Autodesk Inventor part; units mm, degrees
ref_plane "YZ Plane" through (0, 0, 0) normal (1, 0, 0) x (0, 1, 0)
ref_plane "XZ Plane" through (0, 0, 0) normal (0, 1, 0) x (-1, 0, 0)
ref_plane "XY Plane" through (0, 0, 0) normal (0, 0, 1) x (1, 0, 0)
sketch "Sketch1" plane through (0, 0, 0) normal (0, 0, 1) x (1, 0, 0)
  line L0 (0, 0) -> (25.4, 0)
  line L1 (25.4, 76.2) -> (0, 76.2)
  line L2 (0, 76.2) -> (0, 0)
  line L3 (25.4, 3.175) -> (3.175, 3.175)
  line L4 (3.175, 3.175) -> (3.175, 73.025)
  line L5 (3.175, 73.025) -> (25.4, 73.025)
  line L6 (25.4, 0) -> (25.4, 3.175)
  line L7 (25.4, 73.025) -> (25.4, 76.2)
  dimension "d0" = 76.2
  dimension "d1" = 25.4
  dimension "d2" = 3.175
  dimension "d3" = 3.175
  dimension "d4" = 3.175
extrude "Extrusion1" add sketch "Sketch1" along normal blind 685.8
sketch "Sketch2" plane through (0, 76.2, 0) normal (0, 1, 0) x (1, 0, 0)
  line L0 (0, -685.8) -> (25.4, -685.8)
  line L1 (25.4, 0) -> (25.4, -685.8)
  line L2 (25.4, 0) -> (0, 0)
  line L3 (0, 0) -> (0, -685.8)
  line L4 (0, -685.8) -> (25.4, -660.4)
  line L5 (0, 0) -> (25.4, -25.4)
  line L6 (3.175, -682.625) -> (3.175, -517.525)
  line L7 (3.175, -517.525) -> (25.4, -517.525)
  line L8 (3.175, -3.175) -> (3.175, -168.275)
  line L9 (3.175, -168.275) -> (25.4, -168.275)
  dimension "d7" = 45
  dimension "d8" = 3.175
  dimension "d9" = 165.1
  dimension "d10" = 165.1
extrude "Extrusion2" cut sketch "Sketch2" against normal through all contours L4 L1 L0 | L2 L1 L5
extrude "Extrusion3" cut sketch "Sketch2" against normal up to next contours L6 L7 L1 L4 | L5 L1 L9 L8
equation "\"d3\" = d2"
equation "\"d4\" = d2"
equation "\"d10\" = d9"
properties part number "frame U 1 by 3"
Can you work these out from the model? Positions are in its coordinate system, mm. A direction names the side the tool comes from. Round coordinates to 2 decimals unless told otherwise and drop trailing zeros. Order: outer loops, then holes, each group sorted by start corner. A loop starts at its lowest first (then second) coordinate and runs counter-clockwise, first axis right, second up. Notation, with made-up numbers: (80.25, 35) -> (101.25, 35) arc R27 cw to (101.25, 65) -> close; hole circle Ø11 at (47, 67). An arc over 180 degrees is marked (long way). Return JSON: item names as keys, results as strings. Group by question number.
1. If we section it at C-C, the plane y = 27.5: Write out the boundary of the cut face in (x, z) (3 decimals), then the cut area to 3 significant figures.
2. I need wall thicknesses on line 1 (Y direction, x = 12, z = 222.5) (3 decimals); line 2 (X direction, y = 33, z = 478) (3 decimals). Which ranges of each line are inside material? Lowest first, please. Write a range as [from, to].
3. We'd pull the mould along Y, two halves only. Please class faces 3 (the face through (3.175, 40, 348)), 4 (the face through (2, 30, 2)), 5 (the face through (13, 0, 338)): released by +Y, released by -Y, zero draft, split by the parting line, or undercut.
4. Which directions (+Z, -Z, +X, -X, +Y, -Y) give clear straight access to the entire face, cutting with the end or side of a thin tool? Please do faces 1 (the face through (14, 73.025, 340)), 2 (the face through (13, 76.2, 338)).
5. Will these pins go through, and if not, where does the flat tip stop? pin 1 (1.6 mm diameter, centred on x = 17.5, y = 75.5, fed in from -Z) (3 decimals); pin 2 (1.5 mm diameter, centred on y = 12, z = 74, fed in from +X) (3 decimals); pin 3 (3.5 mm diameter, centred on x = 10, y = 75, fed in from +Z) (3 decimals).
6. If we section it at D-D, the plane z = 193: Write out the boundary of the cut face in (x, y) (3 decimals), then the cut area to 3 significant figures.
7. If we section it at B-B, the plane z = 630: Write out the boundary of the cut face in (x, y) (3 decimals), then the cut area to 4 significant figures.
8. If we section it at A-A, the plane x = 20.75: Write out the boundary of the cut face in (y, z) (3 decimals), then the cut area to 3 significant figures.
Output values:
{
 "1": {"outline": "(0, 0) -> (3.175, 3.175) -> (3.175, 682.625) -> (0, 685.8) -> close", "area": "2,170 mm²"},
 "2": {"line 1": "[0, 3.175], [73.025, 76.2]", "line 2": "[0, 3.175]"},
 "3": {"face 3": "undercut", "face 4": "zero draft", "face 5": "released by -Y"},
 "4": {"face 1": "+Z, -Z, +X", "face 2": "+Z, -Z, +X, -X, +Y"},
 "5": {"pin 1": "z = 168.275", "pin 2": "x = 3.175", "pin 3": "z = 517.525"},
 "6": {"outline": "(0, 0) -> (25.4, 0) -> (25.4, 3.175) -> (3.175, 3.175) -> (3.175, 73.025) -> (25.4, 73.025) -> (25.4, 76.2) -> (0, 76.2) -> close", "area": "383 mm²"},
 "7": {"outline": "(0, 0) -> (25.4, 0) -> (25.4, 3.175) -> (3.175, 3.175) -> (3.175, 76.2) -> (0, 76.2) -> close", "area": "312.5 mm²"},
 "8": {"outline": "(0, 20.75) -> (3.175, 20.75) -> (3.175, 665.05) -> (0, 665.05) -> close; (73.025, 168.275) -> (76.2, 168.275) -> (76.2, 517.525) -> (73.025, 517.525) -> close", "area": "3,150 mm²"}
}
